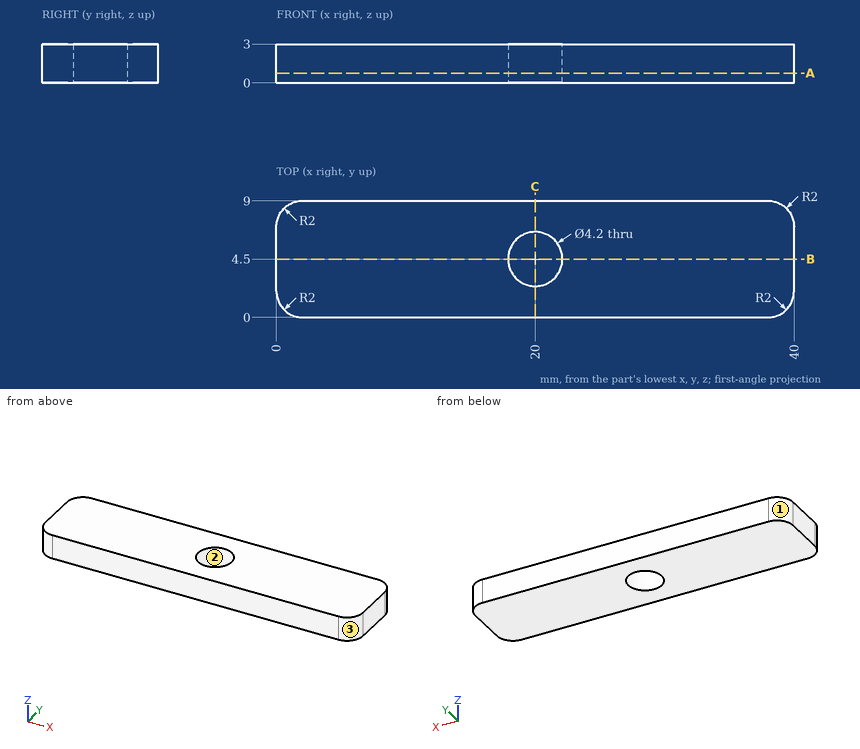
Here's the drawing with two shaded views (mm, measured from the low corner). I have some questions. Coordinates: 2 decimals unless noted, no trailing zeros. Write each loop counter-clockwise with the first axis right and the second up, starting at its lowest first coordinate (ties: lowest second). Pieces come first, ordered by that corner, then holes. Notation, with made-up numbers: M 1.25,-21 L 20.25,-21 A20 ccw 20.25,1 Z; hole C -15.75,57.25 d6. An arc over 180 degrees is marked long. Use one line per item in the form item = value.
Q1. We'd pull the mould along Y, two halves only. Please class the marked faces 1, 2 and 3: +Y half, -Y half, draft (parallel to the pull), parting line (faces both ways), or undercut.
Model answer:
face_1 = +Y half
face_2 = undercut
face_3 = -Y half
Q2. If we section it at B-B (y = 4.5): Write out the boundary of the cut face in (x, z).
Model answer:
outline = M 0,0 L 17.9,0 L 17.9,3 L 0,3 Z; M 22.1,0 L 40,0 L 40,3 L 22.1,3 Z
Q3. If we section it at C-C (x = 20): Write out the boundary of the cut face in (y, z).
Model answer:
outline = M 0,0 L 2.4,0 L 2.4,3 L 0,3 Z; M 6.6,0 L 9,0 L 9,3 L 6.6,3 Z
Q4. I need wall thicknesses on line 1 along Y through (x, z) = (20, 1.5); line 2 along X through (y, z) = (4.75, 1.1); line 3 along X through (y, z) = (0.5, 1.75). Which ranges of each line are inside material? Lowest first, please. Write a range as from..to.
Model answer:
line_1 = 0..2.4, 6.6..9
line_2 = 0..17.91, 22.09..40
line_3 = 0.68..39.32
Q5. If we section it at A-A (z = 0.75): Write out the boundary of the cut face in (x, y), then the cut area to 3 significant figures.
Model answer:
outline = M 0,2 A2 ccw 2,0 L 38,0 A2 ccw 40,2 L 40,7 A2 ccw 38,9 L 2,9 A2 ccw 0,7 Z; hole C 20,4.5 d4.2
area = 343 mm^2
Q6. For P1, Ø3.5, axis at x = 20, y = 4.5, coming from the +Z side, with a flat end and sliding along its axis, tell me the tip position at first contact or that it passes through.
Model answer:
P1 = through
